Could you check a few things on this model? Use its own coordinates, in mm. A direction names the side the tool comes from. Round coordinates to 2 decimals unless told otherwise and drop trailing zeros. Loops run counter-clockwise (first coordinate to the right, second up) from the corner with the lowest first, then second, coordinate; pieces in that order, holes last. Notation, with made-up numbers: (-1.5, 51) -> (12.5, 51) arc R27 cw to (12.5, 80) -> close; hole circle Ø7 at (47.5, -31). An arc over 180 degrees is marked (long way). One line per item, written item: value.
```python
from build123d import *

# Parameters (mm, degrees)
SKETCH1_R                                   = 11.1125
BASE_DEPTH                                  = 4.7625
F_1_4_CAP_SCREW_CARRIAGE_MOUNTS_D           = 6.7564
F_1_4_CAP_SCREW_CARRIAGE_MOUNTS_CBORE_D     = 11.1125
F_1_4_CAP_SCREW_CARRIAGE_MOUNTS_CBORE_DEPTH = 6.35
SKETCH9_R                                   = 2.38125
ALIGNMENT_PIN_HOLES_DEPTH                   = 6.35


with BuildPart() as part:
    # Sketch1 → Base (new, symmetric)
    with BuildSketch(Plane.XY):
        with BuildLine():
            Line((76.2, 11.98626), (76.2, -65.48374))
            Line((76.2, -65.48374), (-76.2, -65.48374))
            Line((-76.2, -65.48374), (-76.2, 11.98626))
            ThreePointArc((-76.2, 11.98626), (-74.340128061, 16.476388061), (-69.85, 18.33626))
            Line((-69.85, 18.33626), (-44.45, 18.33626))
            ThreePointArc((-44.45, 18.33626), (-39.959871939, 16.476388061), (-38.1, 11.98626))
            Line((-38.1, 11.98626), (-38.1, 0))
            ThreePointArc((-38.1, 0), (0, -38.1), (38.1, 0))
            Line((38.1, 0), (38.1, 11.98626))
            ThreePointArc((38.1, 11.98626), (39.959871939, 16.476388061), (44.45, 18.33626))
            Line((44.45, 18.33626), (69.85, 18.33626))
            ThreePointArc((69.85, 18.33626), (74.340128061, 16.476388061), (76.2, 11.98626))
        make_face()
        with Locations(Location((-57.15, 0, 0), (0, 0, 180))):
            Circle(SKETCH1_R, mode=Mode.SUBTRACT)
        with Locations(Location((57.15, 0, 0), (0, 0, 180))):
            Circle(SKETCH1_R, mode=Mode.SUBTRACT)
    extrude(amount=BASE_DEPTH, both=True)

    # 1_4 Cap screw carriage mounts (through all)
    with Locations(Plane(origin=(-61.987391614, 5.409091563, -4.7625), x_dir=(1, 0, 0), z_dir=(0, 0, -1))):
        with Locations((-4.687608386, 51.842831563), (39.762391614, 64.542831563), (128.662391614, 51.842831563), (84.212391614, 64.542831563)):
            CounterBoreHole(F_1_4_CAP_SCREW_CARRIAGE_MOUNTS_D / 2, F_1_4_CAP_SCREW_CARRIAGE_MOUNTS_CBORE_D / 2, F_1_4_CAP_SCREW_CARRIAGE_MOUNTS_CBORE_DEPTH)

    # Sketch9 → Alignment_pin_holes (cut)
    with BuildSketch(Plane(origin=(0, 0, 4.7625), x_dir=(-1, 0, 0), z_dir=(0, 0, -1))):
        with Locations((63.5, -59.13374)):
            Circle(SKETCH9_R)
        with Locations((-63.5, -59.13374)):
            Circle(SKETCH9_R)
    extrude(amount=ALIGNMENT_PIN_HOLES_DEPTH, mode=Mode.SUBTRACT)


solid = part.part
```
Item 1: If we mould it in two halves opening along Y, with no side actions, what happens to faces 1 (the face through (-38.1, 6, 0)), 2 (the face through (68.25, -0.49, -0.07)), 3 (the face through (22.957, -55.836, 3.197)), 4 (the face through (74.29, 16.525, 0.067))? For each: released by +Y, released by -Y, zero draft, split by the parting line, or undercut.
Output:
face 1: zero draft
face 2: undercut
face 3: undercut
face 4: released by +Y
Item 2: If we section it at B-B on y = -23: List the corners of the cut face in (x, z) for me.
Output:
outline: (-76.2, -4.76) -> (-30.37, -4.76) -> (-30.37, 4.76) -> (-76.2, 4.76) -> close; (30.37, -4.76) -> (76.2, -4.76) -> (76.2, 4.76) -> (30.37, 4.76) -> close
Item 3: If we section it at C-C on x = 0: List the corners of the cut face in (y, z) for me.
Output:
outline: (-65.48, -4.76) -> (-38.1, -4.76) -> (-38.1, 4.76) -> (-65.48, 4.76) -> close
Item 4: If we section it at D-D on x = -30: List the corners of the cut face in (y, z) for me, plus the area to 3 significant figures.
Output:
outline: (-65.48, -4.76) -> (-23.49, -4.76) -> (-23.49, 4.76) -> (-65.48, 4.76) -> close
area: 400 mm²
Item 5: I need wall thicknesses on line 1 (X direction, y = -46, z = 0); line 2 (Y direction, x = 57.15, z = -2.5); line 3 (X direction, y = 5.5, z = 3.25). Which ranges of each line are inside material? Lowest first, please. Write a range as from..to.
Output:
line 1: x = -76.2..-72.21, -61.14..61.14, 72.21..76.2
line 2: y = -65.48..-11.11, 11.11..18.34
line 3: x = -76.2..-66.81, -47.49..-38.1, 38.1..47.49, 66.81..76.2
Item 6: Will these pins go through, and if not, where does the flat tip stop? pin 1 Ø9 at (x, y) = (-66.5, -45) entering from -Z; pin 2 Ø3.5 at (x, y) = (19.5, -59.5) entering from -Z; pin 3 Ø1.4 at (x, y) = (63.5, -58.5) entering from +Z.
Output:
pin 1: stops at z = -4.76
pin 2: stops at z = 1.59
pin 3: stops at z = -1.59
Item 7: For faces 5 (the face through (39.911, 16.427, 0.067)), 6 (the face through (-62.984, -61.458, 1.632)), 7 (the face through (63.453, -47.448, 3.197)), 8 (the face through (-57, 18.336, 0)), 9 (the face through (-64, -44, 1.587)), which set-ups out of +Z, -Z, +X, -X, +Y, -Y let a thin tool reach every point of the face, with its end or its side?
Output:
face 5: +Z, -Z, +Y
face 6: +Z
face 7: +Z, -Z
face 8: +Z, -Z, +X, -X, +Y
face 9: -Z
Item 8: If we section it at A-A on x = 57.15: List the corners of the cut face in (y, z) for me.
Output:
outline: (-65.48, -4.76) -> (-11.11, -4.76) -> (-11.11, 4.76) -> (-65.48, 4.76) -> close; (11.11, -4.76) -> (18.34, -4.76) -> (18.34, 4.76) -> (11.11, 4.76) -> close
